Can you work these out from the model? Positions are in its coordinate system, mm. Coordinates: 2 decimals unless noted, no trailing zeros. Write each loop counter-clockwise with the first axis right and the second up, starting at its lowest first coordinate (ties: lowest second). Pieces come first, ordered by that corner, then holes. Notation, with made-up numbers: (3.25, 67) -> (62.25, 67) arc R26 cw to (62.25, 81) -> close; hole circle Ø11 at (-22, -6.5). An arc over 180 degrees is marked (long way). Answer as CSV lines item,"result". Start each with the question number.
```python
from build123d import *

# Parameters (mm, degrees)
BOSS_EXTRUDE1_DEPTH = 15
SKETCH2_R           = 2.5
CUT_EXTRUDE1_DEPTH  = 15


with BuildPart() as part:
    # Sketch1 → Boss-Extrude1 (new body)
    with BuildSketch(Plane.XY):
        with BuildLine():
            ThreePointArc((5, 40), (0, 35), (-5, 40))
            Line((-5, 40), (-5, -40))
            ThreePointArc((-5, -40), (0, -35), (5, -40))
            Line((5, -40), (5, 40))
        make_face()
        with BuildLine():
            ThreePointArc((5, 40), (0, 45), (-5, 40))
            Line((-5, 40), (5, 40))
        make_face()
        with BuildLine():
            Line((5, 40), (-5, 40))
            ThreePointArc((-5, 40), (0, 35), (5, 40))
        make_face()
        with BuildLine():
            ThreePointArc((5, -40), (0, -35), (-5, -40))
            Line((-5, -40), (5, -40))
        make_face()
        with BuildLine():
            Line((5, -40), (-5, -40))
            ThreePointArc((-5, -40), (0, -45), (5, -40))
        make_face()
    extrude(amount=BOSS_EXTRUDE1_DEPTH)

    # Sketch2 → Cut-Extrude1 (cut)
    with BuildSketch(Plane.XY.offset(15)):
        with Locations((0, 40)):
            Circle(SKETCH2_R)
        with Locations((0, -40)):
            Circle(SKETCH2_R)
    extrude(amount=-CUT_EXTRUDE1_DEPTH, mode=Mode.SUBTRACT)


solid = part.part
```
Q1. I need wall thicknesses on L1, parallel to Y at x = 0, z = 7.75; L2, parallel to Y at x = -1, z = 4; L3, parallel to Y at x = 3.5, z = 6.5. Which ranges of each line are inside material? Lowest first, please.
Q2. If we mould it in two halves opening along X, with no side actions, what happens to faces 1 (the face through (-0.54, 37.56, 7.6)), 2 (the face through (0, 1, 0)), 3 (the face through (5, -1, 7))? For each: released by +X, released by -X, zero draft, split by the parting line, or undercut.
Q3. Imagine slicing it at B-B (z = 3.5). Write out the boundary of the cut face in (x, y).
Q4. Imagine slicing it at C-C (x = -3.5). Write out the boundary of the cut face in (y, z), then the cut area to 3 significant figures.
Q5. For pin 1 (5 mm diameter, centred on x = -3.5, z = 6, fed in from -Y), with a flat end and sliding along its axis, tell me the tip position at first contact or that it passes through.
Q6. Imagine slicing it at A-A (x = 0). Write out the boundary of the cut face in (y, z), then the cut area to 3 significant figures.
Entries:
1,L1,"-45 to -42.5, -37.5 to 37.5, 42.5 to 45"
1,L2,"-44.9 to -42.29, -37.71 to 37.71, 42.29 to 44.9"
1,L3,"-43.57 to 43.57"
2,face 1,"undercut"
2,face 2,"zero draft"
2,face 3,"released by +X"
3,outline,"(-5, -40) arc R5 ccw to (5, -40) -> (5, 40) arc R5 ccw to (-5, 40) -> close; hole circle Ø5 at (0, -40); hole circle Ø5 at (0, 40)"
4,outline,"(-43.57, 0) -> (43.57, 0) -> (43.57, 15) -> (-43.57, 15) -> close"
4,area,"1,310 mm2"
5,pin 1,"y = -44.9"
6,outline,"(-45, 0) -> (-42.5, 0) -> (-42.5, 15) -> (-45, 15) -> close; (-37.5, 0) -> (37.5, 0) -> (37.5, 15) -> (-37.5, 15) -> close; (42.5, 0) -> (45, 0) -> (45, 15) -> (42.5, 15) -> close"
6,area,"1,200 mm2"
